Input: part model. Units: mm. Frame: model coordinates. Face numbers are marked on the shaded views. A direction names the side the tool comes from. Coordinates: 2 decimals unless noted, no trailing zeros. Write each loop counter-clockwise with the first axis right and the second up, starting at its lowest first coordinate (ties: lowest second). Pieces come first, ordered by that corner, then holes. Notation, with made-up numbers: (3, -15) - (12, -15) arc R23 cw to (12, 0) - close; hole circle Ø3 at (-15.5, 0.5). An arc over 180 degrees is marked (long way). Use CSV: the item, a comma, the result in double quotes.
```python
from build123d import *

# Parameters (mm, degrees)
SKETCH2_W           = 100
SKETCH2_H           = 90
SKETCH2_R           = 1.5
BOSS_EXTRUDE1_DEPTH = 8
SKETCH5_W           = 100
SKETCH5_H           = 10
BOSS_EXTRUDE2_DEPTH = 35
SKETCH7_R           = 7.5
SKETCH7_R_2         = 3.75
CUT_EXTRUDE2_DEPTH  = 290


with BuildPart() as part:
    # Sketch2 → Boss-Extrude1 (new body)
    with BuildSketch(Plane.XY):
        Rectangle(SKETCH2_W, SKETCH2_H)
        with Locations(Location((-9, -4.165902831, 0), (0, 0, 180))):
            Circle(SKETCH2_R, mode=Mode.SUBTRACT)
        with Locations(Location((9, -28.094631071, 0), (0, 0, 180))):
            Circle(SKETCH2_R, mode=Mode.SUBTRACT)
        with Locations((9, -4.165902831)):
            Circle(SKETCH2_R, mode=Mode.SUBTRACT)
        with Locations((-9, -28.094631071)):
            Circle(SKETCH2_R, mode=Mode.SUBTRACT)
        with Locations(Location((-9, 28.094631071, 0), (0, 0, 180))):
            Circle(SKETCH2_R, mode=Mode.SUBTRACT)
        with Locations((9, 28.094631071)):
            Circle(SKETCH2_R, mode=Mode.SUBTRACT)
        with Locations(Location((9, 4.165902831, 0), (0, 0, 180))):
            Circle(SKETCH2_R, mode=Mode.SUBTRACT)
        with Locations((-9, 4.165902831)):
            Circle(SKETCH2_R, mode=Mode.SUBTRACT)
    extrude(amount=BOSS_EXTRUDE1_DEPTH)

    # Sketch5 → Boss-Extrude2 (add)
    with BuildSketch(Plane.XY.offset(8)):
        with Locations((0, 40)):
            Rectangle(SKETCH5_W, SKETCH5_H)
        with Locations((0, -40)):
            Rectangle(SKETCH5_W, SKETCH5_H)
    extrude(amount=BOSS_EXTRUDE2_DEPTH)

    # Sketch7 → Cut-Extrude2 (cut)
    with BuildSketch(Plane(origin=(0, 45, 0), x_dir=(1, 0, 0), z_dir=(0, 1, 0))):
        with Locations(Location((-3.365, -21.5, 0), (0, 0, 270))):
            Circle(SKETCH7_R)
        with Locations(Location((-40.365, -21.5, 0), (0, 0, 270))):
            Circle(SKETCH7_R_2)
        with Locations(Location((33.635, -21.5, 0), (0, 0, 270))):
            Circle(SKETCH7_R_2)
    extrude(amount=-CUT_EXTRUDE2_DEPTH, mode=Mode.SUBTRACT)


solid = part.part
```
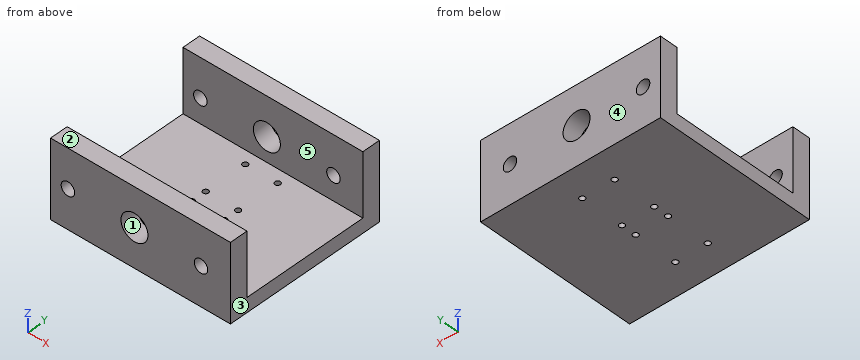
(1) Reachability of the marked faces 4 and 5 from +Z, -Z, +X, -X, +Y, -Y: full face, straight path, thin tool, end or side. Return the list, or none.
Check values:
face 4,"+Z, -Z, +X, -X, +Y"
face 5,"+Z, +X, -X"
(2) Cut plane B-B on x = 9. Return loops of the section in (y, z), and give its area (3 significant figures).
Check values:
outline,"(-45, 0) - (-29.59, 0) - (-29.59, 8) - (-35, 8) - (-35, 43) - (-45, 43) - close; (-26.59, 0) - (-5.67, 0) - (-5.67, 8) - (-26.59, 8) - close; (-2.67, 0) - (2.67, 0) - (2.67, 8) - (-2.67, 8) - close; (5.67, 0) - (26.59, 0) - (26.59, 8) - (5.67, 8) - close; (29.59, 0) - (45, 0) - (45, 43) - (35, 43) - (35, 8) - (29.59, 8) - close"
area,"1,320 mm^2"
(3) Cut plane A-A on z = 11.5. Return loops of the section in (x, y), and give its area (3 significant figures).
Check values:
outline,"(-50, -45) - (50, -45) - (50, -35) - (-50, -35) - close; (-50, 35) - (50, 35) - (50, 45) - (-50, 45) - close"
area,"2,000 mm^2"
(4) Ray query, probe 1 along Y at (x, z) = (9, 5); probe 2 along Y at (x, z) = (22, 29.5); probe 3 along Z at (x, y) = (-13.5, -19). Return the intervals inside material, ascending. Write a range as from..to.
Check values:
probe 1,"-45..-29.59, -26.59..-5.67, -2.67..2.67, 5.67..26.59, 29.59..45"
probe 2,"-45..-35, 35..45"
probe 3,"0..8"
(5) Cut plane D-D on x = 40. Return loops of the section in (y, z).
Check values:
outline,"(-45, 0) - (45, 0) - (45, 43) - (35, 43) - (35, 8) - (-35, 8) - (-35, 43) - (-45, 43) - close"
(6) Cut plane C-C on z = 21.5. State how many separate pieces and enclosed holes the cut face has, and give its area (3 significant figures).
Check values:
separate pieces,"8"
enclosed holes,"0"
area,"1,400 mm^2"
(7) Draft query along Z for the marked faces 1, 2 and 3. Return one class per face: pulls with the +Z half, pulls with the -Z half, needs draft (parallel to the pull), parting line crosses it, or undercut.
Check values:
face 1,"undercut"
face 2,"pulls with the +Z half"
face 3,"needs draft"
(8) Pin query (flat end, axial travel): pin 1 Ø2.5 at (x, y) = (9, 28.09) entering from -Z; pin 2 Ø21 at (x, y) = (16, 3) entering from +Z. Return the tip coordinate at first contact, or that it passes through.
Check values:
pin 1,"through"
pin 2,"z = 8"
